For this review, take the finished solid that the model builds, in its own axes (mm). Face numbers are marked on the shaded views. A direction names the side the tool comes from. Round coordinates to 2 decimals unless told otherwise and drop trailing zeros. Loops run counter-clockwise (first coordinate to the right, second up) from the corner with the lowest first, then second, coordinate; pieces in that order, holes last. Notation, with made-up numbers: (45, 32) -> (98, 32) arc R16 ccw to (98, 59) -> close; hole circle Ø10 at (5.25, 66.5). An arc over 180 degrees is marked (long way). One line per question, with ' | ' between items. Start each with the question number.
1. Wall thickness on line 1 along Z through (x, y) = (11, 9.5); line 2 along X through (y, z) = (27.5, -18); line 3 along X through (y, z) = (-1.15, 59): over which ranges is each line inside the solid? List them lowest first.
2. For the marked faces 5 and 6, list the 3-axis set-ups (+Z, -Z, +X, -X, +Y, -Y) from which the entire face can be reached by the end or side of a thin tool; tool diameter is ignored.
3. For pin 1 Ø13 at (x, y) = (-15, 15.5) entering from -Z; pin 2 Ø20 at (x, y) = (2.5, 14.5) entering from +Z; pin 3 Ø14.5 at (x, z) = (36.5, -60.5) entering from +Y, all flat-tipped, find the tip position at first contact; note any pin that passes through.
4. Consider section D-D (x = 18). Write out the cut boundary in (y, z).
5. Draft analysis for pull direction Z (two halves, no side actions). For the marked faces 1, 2, 3 and 4, state which applies: pulls with the +Z half, pulls with the -Z half, needs draft (parallel to the pull), parting line crosses it, or undercut.
6. Consider section C-C (z = 45). Write out the cut boundary in (x, y).
7. Consider section B-B (y = 33). Write out the cut boundary in (x, z), and give its area (3 significant figures).
8. Consider section A-A (x = 43). Write out the cut boundary in (y, z).
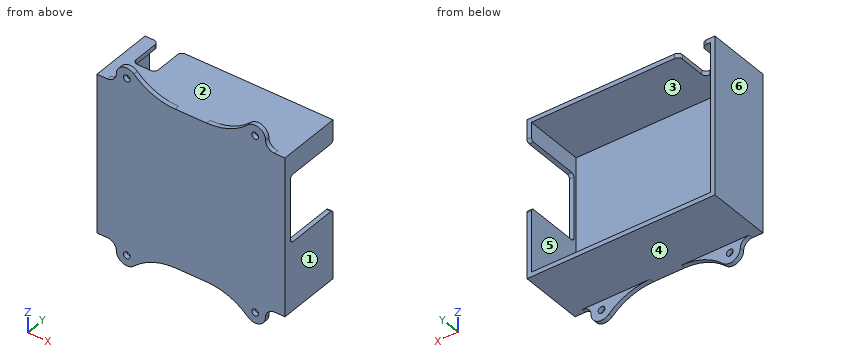
```python
from build123d import *

# Parameters (mm, degrees)
SKETCH1_W           = 126
SKETCH1_H           = 106
SKETCH1_W_2         = 120
SKETCH1_H_2         = 100
BOSS_EXTRUDE1_DEPTH = 40
SKETCH2_R           = 2.25
BOSS_EXTRUDE2_DEPTH = 3
SKETCH3_W           = 15
SKETCH3_H           = 23
CUT_EXTRUDE1_DEPTH  = 3
FILLET1_R           = 3
SKETCH4_W           = 45
SKETCH4_H           = 38
CUT_EXTRUDE2_DEPTH  = 3
FILLET2_R           = 2


with BuildPart() as part:
    # Sketch1 → Boss-Extrude1 (new body)
    with BuildSketch(Plane(origin=(0, 0, 0), x_dir=(1, 0, 0), z_dir=(0, 1, 0))):
        Rectangle(SKETCH1_W, SKETCH1_H)
        Rectangle(SKETCH1_W_2, SKETCH1_H_2, mode=Mode.SUBTRACT)
    extrude(amount=BOSS_EXTRUDE1_DEPTH)

    # Sketch2 → Boss-Extrude2 (add)
    with BuildSketch(Plane.XZ):
        with BuildLine():
            Line((56, 53), (63, 53))
            Line((63, 53), (63, -53))
            Line((63, -53), (56, -53))
            ThreePointArc((56, -53), (51.757359313, -54.757359313), (50, -59))
            ThreePointArc((50, -59), (45.754014261, -65.435480204), (38.167027014, -64.063829787))
            ThreePointArc((38.167027014, -64.063829787), (25.425407281, -55.868835135), (10.550038521, -53))
            Line((10.550038521, -53), (-10.550038521, -53))
            ThreePointArc((-10.550038521, -53), (-25.425407281, -55.868835135), (-38.167027014, -64.063829787))
            ThreePointArc((-38.167027014, -64.063829787), (-45.754014261, -65.435480204), (-50, -59))
            ThreePointArc((-50, -59), (-51.757359313, -54.757359313), (-56, -53))
            Line((-56, -53), (-63, -53))
            Line((-63, -53), (-63, 53))
            Line((-63, 53), (-56, 53))
            ThreePointArc((-56, 53), (-51.757359313, 54.757359313), (-50, 59))
            ThreePointArc((-50, 59), (-45.754014261, 65.435480204), (-38.167027014, 64.063829787))
            ThreePointArc((-38.167027014, 64.063829787), (-25.425407281, 55.868835135), (-10.550038521, 53))
            Line((-10.550038521, 53), (10.550038521, 53))
            ThreePointArc((10.550038521, 53), (25.425407281, 55.868835135), (38.167027014, 64.063829787))
            ThreePointArc((38.167027014, 64.063829787), (45.754014261, 65.435480204), (50, 59))
            ThreePointArc((50, 59), (51.757359313, 54.757359313), (56, 53))
        make_face()
        with Locations(Location((43, 59, 0), (0, 0, 270))):
            Circle(SKETCH2_R, mode=Mode.SUBTRACT)
        with Locations(Location((43, -59, 0), (0, 0, 90))):
            Circle(SKETCH2_R, mode=Mode.SUBTRACT)
        with Locations(Location((-43, -59, 0), (0, 0, 270))):
            Circle(SKETCH2_R, mode=Mode.SUBTRACT)
        with Locations(Location((-43, 59, 0), (0, 0, 90))):
            Circle(SKETCH2_R, mode=Mode.SUBTRACT)
    extrude(amount=BOSS_EXTRUDE2_DEPTH)

    # Sketch3 → Cut-Extrude1 (cut)
    with BuildSketch(Plane.XY.offset(53)):
        with Locations((-46.5, 28.5)):
            Rectangle(SKETCH3_W, SKETCH3_H)
    extrude(amount=-CUT_EXTRUDE1_DEPTH, mode=Mode.SUBTRACT)

    # Fillet1
    fillet1_edges = [part.edges().sort_by_distance(p)[0] for p in [
        (-54, 17, 51.5),
        (-54, 40, 51.5),
        (-39, 40, 51.5),
        (-39, 17, 51.5),
    ]]
    fillet(fillet1_edges, radius=FILLET1_R)

    # Sketch4 → Cut-Extrude2 (cut)
    with BuildSketch(Plane(origin=(63, 0, 0), x_dir=(0, 0, -1), z_dir=(1, 0, 0))):
        with Locations((-15.5, 21)):
            Rectangle(SKETCH4_W, SKETCH4_H)
    extrude(amount=-CUT_EXTRUDE2_DEPTH, mode=Mode.SUBTRACT)

    # Fillet2
    fillet2_edges = [part.edges().sort_by_distance(p)[0] for p in [
        (61.5, 2, 38),
        (61.5, 40, 38),
        (61.5, 40, -7),
        (61.5, 2, -7),
    ]]
    fillet(fillet2_edges, radius=FILLET2_R)


solid = part.part
```
Answer block:
1) line 1: z = -53 to -50, 50 to 53 | line 2: x = -63 to -60, 60 to 63 | line 3: x = -50 to -45.25, -40.75 to -31.62, 31.62 to 40.75, 45.25 to 50
2) face 5: +Y | face 6: +Z, -Z, -X, +Y, -Y
3) pin 1: stops at z = -53 | pin 2: stops at z = 53 | pin 3: stops at y = 0
4) outline: (-3, -53.7) -> (0, -53.7) -> (0, -53) -> (40, -53) -> (40, -50) -> (0, -50) -> (0, 50) -> (40, 50) -> (40, 53) -> (0, 53) -> (0, 53.7) -> (-3, 53.7) -> close
5) face 1: needs draft | face 2: pulls with the +Z half | face 3: undercut | face 4: pulls with the -Z half
6) outline: (-63, -3) -> (63, -3) -> (63, 40) -> (60, 40) -> (60, 0) -> (-60, 0) -> (-60, 40) -> (-63, 40) -> close
7) outline: (-63, -53) -> (63, -53) -> (63, -7) -> (60, -7) -> (60, -50) -> (-60, -50) -> (-60, 50) -> (-54, 50) -> (-54, 53) -> (-63, 53) -> close; (-39, 50) -> (60, 50) -> (60, 38) -> (63, 38) -> (63, 53) -> (-39, 53) -> close | area: 1,180 mm2
8) outline: (-3, -66) -> (0, -66) -> (0, -61.25) -> (-3, -61.25) -> close; (-3, -56.75) -> (0, -56.75) -> (0, -53) -> (40, -53) -> (40, -50) -> (0, -50) -> (0, 50) -> (40, 50) -> (40, 53) -> (0, 53) -> (0, 56.75) -> (-3, 56.75) -> close; (-3, 61.25) -> (0, 61.25) -> (0, 66) -> (-3, 66) -> close
